Can you work these out from the model? Positions are in its coordinate system, mm. Face numbers are marked on the shaded views. A direction names the side the tool comes from. Give positions to 0.01 mm unless a question says otherwise; leave off trailing zeros. Write each loop counter-clockwise with the first axis right and the second up, starting at its lowest first coordinate (ties: lowest second). Pieces come first, ordered by that corner, then holes.
```python
from build123d import *

# Parameters (mm, degrees)
SKETCH_1_W                = 40
SKETCH_1_H                = 40
EXTRUDE_1_DEPTH           = 4
SKETCH_2_W                = 40
SKETCH_2_H                = 4
EXTRUDE_2_DEPTH           = 4
SKETCH_3_W                = 40
SKETCH_3_H                = 4
EXTRUDE_3_DEPTH           = 20
SKETCH_4_W                = 8
SKETCH_4_H                = 12
EXTRUDE_4_DEPTH           = 4
CUT_EXTRUDE_1_DEPTH       = 11
EXTRUDE_5_DEPTH           = 4
EXTRUDE_6_DEPTH           = 4
EXTRUDE_7_DEPTH           = 4
SKETCH_10_W               = 23
SKETCH_10_H               = 24.293070416
EXTRUDE_8_DEPTH           = 10
CUT_EXTRUDE_3_DEPTH       = 25.293070415
SKETCH_14_W               = 8
SKETCH_14_H               = 0.5
CUT_EXTRUDE_4_DEPTH       = 45
SKETCH_15_W               = 23
SKETCH_15_H               = 1
CUT_EXTRUDE_5_DEPTH       = 45
SKETCH_16_R               = 2.6
CUT_EXTRUDE_6_DEPTH       = 7
SKETCH_17_W               = 52
SKETCH_17_H               = 4
CUT_EXTRUDE_7_DEPTH       = 20
CUT_EXTRUDE_8_DEPTH       = 0.29
SKETCH_20_R               = 1
CUT_EXTRUDE_9_DEPTH       = 11
CUT_EXTRUDE_10_DEPTH      = 1
CUT_EXTRUDE_10_DEPTH_BACK = 4
FILLET_1_R                = 1


with BuildPart() as part:
    # 草图1 → 凸台-拉伸1 (new body)
    with BuildSketch(Plane.XY):
        with Locations((-0.053475936, -8.663101604)):
            Rectangle(SKETCH_1_W, SKETCH_1_H)
    extrude(amount=EXTRUDE_1_DEPTH)

    # 草图2 → 凸台-拉伸2 (add)
    with BuildSketch(Plane(origin=(0, 11.336898396, 0), x_dir=(1, 0, 0), z_dir=(0, 1, 0))):
        with Locations((-0.053475936, -2)):
            Rectangle(SKETCH_2_W, SKETCH_2_H)
    extrude(amount=EXTRUDE_2_DEPTH)

    # 草图3 → 凸台-拉伸3 (add)
    with BuildSketch(Plane(origin=(0, 0, 0), x_dir=(-1, 0, 0), z_dir=(0, 0, -1))):
        with Locations((0.053475936, 13.336898396)):
            Rectangle(SKETCH_3_W, SKETCH_3_H)
    extrude(amount=EXTRUDE_3_DEPTH)

    # 草图4 → 凸台-拉伸4 (add)
    with BuildSketch(Plane.XY.offset(4)):
        with Locations((-10.534642548, 9.336898396)):
            Rectangle(SKETCH_4_W, SKETCH_4_H)
    extrude(amount=EXTRUDE_4_DEPTH)

    # 草图6 → 切除-拉伸1 (cut)
    with BuildSketch(Plane(origin=(0, 15.336898396, 0), x_dir=(1, 0, 0), z_dir=(0, 1, 0))):
        with BuildLine():
            Line((-8.534642548, -8), (-12.534642548, -8))
            ThreePointArc((-12.534642548, -8), (-10.534642548, -6), (-8.534642548, -8))
        make_face()
    extrude(amount=-CUT_EXTRUDE_1_DEPTH, mode=Mode.SUBTRACT)

    # 草图8 → 凸台-拉伸5 (add)
    with BuildSketch(Plane.ZY.offset(20.053475936)):
        Polygon((4, 15.336898396), (-20, 15.336898396), (-20, 11.336898396), (0, 11.336898396), (0, -28.663101604), (4, -28.663101604), align=None)
    extrude(amount=EXTRUDE_5_DEPTH)

    # 草图9 → 凸台-拉伸6 (add)
    with BuildSketch(Plane(origin=(19.946524064, 0, 0), x_dir=(0, 0, -1), z_dir=(1, 0, 0))):
        Polygon((0, -28.663101604), (0, 11.336898396), (20, 11.336898396), (20, 15.336898396), (-4, 15.336898396), (-4, -28.663101604), align=None)
    extrude(amount=EXTRUDE_6_DEPTH)

    # 草图11 → 凸台-拉伸7 (add)
    with BuildSketch(Plane(origin=(23.946524064, 0, 0), x_dir=(0, 0, -1), z_dir=(1, 0, 0))):
        Polygon((-4, -28.663101604), (0, -28.663101604), (0, 11.336898396), (20, 11.336898396), (20, 15.336898396), (-4, 15.336898396), align=None)
    extrude(amount=EXTRUDE_7_DEPTH)

    # 草图10 → 凸台-拉伸8 (add)
    with BuildSketch(Plane.XY.offset(4)):
        with Locations((12.007361252, 3.190363188)):
            Rectangle(SKETCH_10_W, SKETCH_10_H)
    extrude(amount=EXTRUDE_8_DEPTH)

    # 草图12 → 切除-拉伸3 (cut, through all)
    with BuildSketch(Plane.XZ.offset(8.95617202)):
        with BuildLine():
            Line((4.507361252, 14), (19.507361252, 14))
            ThreePointArc((19.507361252, 14), (12.007361252, 6.5), (4.507361252, 14))
        make_face()
    extrude(amount=-CUT_EXTRUDE_3_DEPTH, mode=Mode.SUBTRACT)

    # 草图14 → 切除-拉伸4 (cut, through all)
    with BuildSketch(Plane(origin=(0, 15.336898396, 0), x_dir=(1, 0, 0), z_dir=(0, 1, 0))):
        with Locations((-10.534642548, -7.75)):
            Rectangle(SKETCH_14_W, SKETCH_14_H)
    extrude(amount=-CUT_EXTRUDE_4_DEPTH, mode=Mode.SUBTRACT)

    # 草图15 → 切除-拉伸5 (cut, through all)
    with BuildSketch(Plane(origin=(0, 15.336898396, 0), x_dir=(1, 0, 0), z_dir=(0, 1, 0))):
        with Locations((12.007361252, -13.5)):
            Rectangle(SKETCH_15_W, SKETCH_15_H)
    extrude(amount=-CUT_EXTRUDE_5_DEPTH, mode=Mode.SUBTRACT)

    # 草图16 → 切除-拉伸6 (cut)
    with BuildSketch(Plane(origin=(0, 15.336898396, 0), x_dir=(1, 0, 0), z_dir=(0, 1, 0))):
        with Locations((-11.053475936, 10)):
            Circle(SKETCH_16_R)
        with Locations((14.946524064, 10)):
            Circle(SKETCH_16_R)
    extrude(amount=-CUT_EXTRUDE_6_DEPTH, mode=Mode.SUBTRACT)

    # 草图17 → 切除-拉伸7 (cut)
    with BuildSketch(Plane.XZ.offset(28.663101604)):
        with Locations((1.946524064, 2)):
            Rectangle(SKETCH_17_W, SKETCH_17_H)
    extrude(amount=-CUT_EXTRUDE_7_DEPTH, mode=Mode.SUBTRACT)

    # 草图19 → 切除-拉伸8 (cut)
    with BuildSketch(Plane.XZ.offset(8.95617202)):
        with BuildLine():
            Line((23.507361252, 4), (23.507361252, 13))
            Line((23.507361252, 13), (19.440395626, 13))
            ThreePointArc((19.440395626, 13), (12.007361252, 6.5), (4.574326878, 13))
            Line((4.574326878, 13), (0.507361252, 13))
            Line((0.507361252, 13), (0.507361252, 4))
            Line((0.507361252, 4), (23.507361252, 4))
        make_face()
    extrude(amount=-CUT_EXTRUDE_8_DEPTH, mode=Mode.SUBTRACT)

    # 草图20 → 切除-拉伸9 (cut)
    with BuildSketch(Plane(origin=(0, 3.336898396, 0), x_dir=(-1, 0, 0), z_dir=(0, -1, 0))):
        with Locations((10.534642548, -7.5)):
            Circle(SKETCH_20_R)
    extrude(amount=-CUT_EXTRUDE_9_DEPTH, mode=Mode.SUBTRACT)

    # 草图21 → 切除-拉伸10 (cut, two sides)
    with BuildSketch(Plane(origin=(0, 15.336898396, 0), x_dir=(1, 0, 0), z_dir=(0, 1, 0))) as cut_extrude_10_sk:
        Polygon((152.48909257, -4), (27.946524064, -4), (-24.053475936, -4), (-148.596044442, -4), (-148.596044442, -253.085137012), (152.48909257, -253.085137012), align=None)
    extrude(amount=CUT_EXTRUDE_10_DEPTH, mode=Mode.SUBTRACT)
    extrude(cut_extrude_10_sk.sketch, amount=-CUT_EXTRUDE_10_DEPTH_BACK, mode=Mode.SUBTRACT)

    # 圆角1
    fillet_1_edges = [part.edges().sort_by_distance(p)[0] for p in [
        (1.946524064, 15.336898396, 4),
        (-24.053475936, 15.336898396, -8),
        (27.946524064, 15.336898396, -8),
    ]]
    fillet(fillet_1_edges, radius=FILLET_1_R)


solid = part.part
```
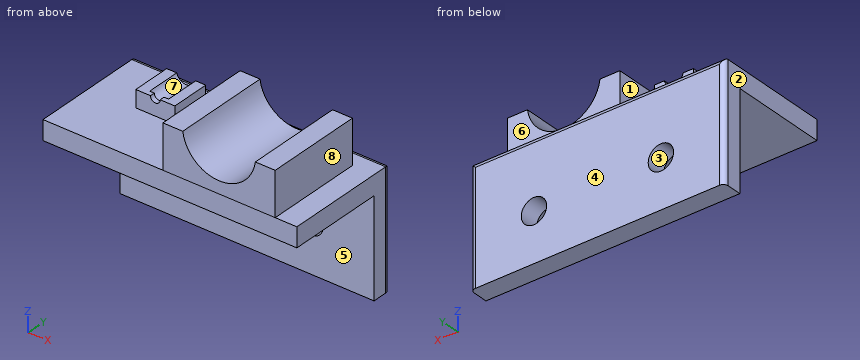
1) Suppose I cut it at C-C on z = 10. Write out the boundary of the cut face in (x, y), plus the area to 3 significant figures.
Values follow:
outline: (0.51, -8.67) - (5.66, -8.67) - (5.66, 11.34) - (0.51, 11.34) - close; (18.35, -8.67) - (23.51, -8.67) - (23.51, 11.34) - (18.35, 11.34) - close
area: 206 mm2
2) Please list where these lines run through material, in increasing order: L1, parallel to X at y = 14.1, z = -10; L2, parallel to X at y = 13.5, z = -12; L3, parallel to Z at x = -5.5, y = -4.75.
Values follow:
L1: x = -24.05 to -13.65, -8.45 to 12.35, 17.55 to 27.95
L2: x = -24.05 to -12.71, -9.39 to 13.29, 16.61 to 27.95
L3: z = 0 to 4
3) For pin 1 Ø4 at (y, z) = (3, 9) entering from +X; pin 2 Ø6 at (x, z) = (12, -11) entering from -Y; pin 3 Ø3 at (x, z) = (-10.5, 6.5) entering from +Y; pin 4 Ø4 at (x, z) = (-11.05, -10) entering from -Y, each with a flat end and sliding along its axis, tell me the tip position at first contact or that it passes through.
Values follow:
pin 1: stops at x = 23.51
pin 2: stops at y = 11.34
pin 3: stops at y = 11.34
pin 4: passes through
4) If we mould it in two halves opening along X, with no side actions, what happens to the marked faces 1, 2, 3 and 4? For each: +X half, -X half, draft (parallel to the pull), parting line (faces both ways), or undercut.
Values follow:
face 1: undercut
face 2: -X half
face 3: undercut
face 4: draft
5) For the marked faces 5, 6, 7 and 8, which set-ups out of +Z, -Z, +X, -X, +Y, -Y let a thin tool reach every point of the face, with its end or its side?
Values follow:
face 5: -Z, +X, -X, -Y
face 6: +Z, +X, -X, +Y
face 7: +Z, +Y
face 8: +Z, +X, +Y, -Y
6) Suppose I cut it at A-A on z = -10. Write out the boundary of the cut face in (x, y).
Values follow:
outline: (-24.05, 11.34) - (-13.65, 11.34) - (-13.65, 15.34) - (-23.05, 15.34) arc R1 ccw to (-24.05, 14.34) - close; (-8.45, 11.34) - (12.35, 11.34) - (12.35, 15.34) - (-8.45, 15.34) - close; (17.55, 11.34) - (27.95, 11.34) - (27.95, 14.34) arc R1 ccw to (26.95, 15.34) - (17.55, 15.34) - close
7) Suppose I cut it at D-D on y = -2.25. Write out the boundary of the cut face in (x, z).
Values follow:
outline: (-24.05, 0) - (27.95, 0) - (27.95, 4) - (23.51, 4) - (23.51, 13) - (19.44, 13) arc R7.5 cw to (4.57, 13) - (0.51, 13) - (0.51, 4) - (-24.05, 4) - close
